from build123d import *

# Parameters (mm, degrees)
F0_W     = 101.6
F0_H     = 152.4
F0_H_2   = 101.6
F1_DEPTH = 152.4
F2_W     = 101.6
F2_H     = 101.6
F3_DEPTH = 228.601
F4_R     = 25.4
F5_DEPTH = 152.401


with BuildPart() as f1:
    # F0 (on Top) → F1 (new body)
    with BuildSketch(Plane.XY):
        with Locations((50.8, 76.2)):
            Rectangle(F0_W, F0_H)
        with Locations((50.8, -50.8)):
            Rectangle(F0_W, F0_H_2)
        Polygon((-76.2, 254), (0, 152.4), (101.6, 152.4), (25.4, 254), align=None)
        Polygon((-127, 304.8), (-76.2, 254), (25.4, 254), align=None)
    extrude(amount=F1_DEPTH)

    # F2 (on face) → F3 (cut, through all)
    with BuildSketch(Plane.YZ.offset(101.6)):
        with Locations((-50.8, 76.2)):
            Rectangle(F2_W, F2_H)
    extrude(amount=-F3_DEPTH, mode=Mode.SUBTRACT)

    # F4 (on face) → F5 (cut, through all)
    with BuildSketch(Plane.XY.offset(152.4)):
        with Locations((50.8, -50.8)):
            Circle(F4_R)
        with BuildLine():
            ThreePointArc((101.6, -50.8), (86.721024, -86.721024), (50.8, -101.6))
            Line((50.8, -101.6), (101.6, -101.6))
            Line((101.6, -101.6), (101.6, -50.8))
        make_face()
        with BuildLine():
            ThreePointArc((50.8, -101.6), (14.878976, -86.721024), (0, -50.8))
            Line((0, -50.8), (0, -101.6))
            Line((0, -101.6), (50.8, -101.6))
        make_face()
    extrude(amount=-F5_DEPTH, mode=Mode.SUBTRACT)


solid = f1.part
Source: CAD feature listing. Evaluate the final solid. Frame: model axes, mm. A direction names the side the tool comes from. Give positions to 0.01 mm unless a question says otherwise; leave off trailing zeros. Write each loop counter-clockwise with the first axis right and the second up, starting at its lowest first coordinate (ties: lowest second). Pieces come first, ordered by that corner, then holes. Notation, with made-up numbers: M -24,88 L -2,88 A12 cw -2,97 Z; hole C 3,-1 d4. An arc over 180 degrees is marked long. Return JSON: item names as keys, results as strings. Group by question number.
1) Cut plane A-A, the plane z = 131. Output: boundary loops of the cut face in (x, y).
2) First-contact query: pin 1 Ø8 at (x, z) = (19, 86.5) entering from -Y; pin 2 Ø12 at (x, z) = (-69, 92) entering from +Y; pin 3 Ø1.5 at (y, z) = (88, 19) entering from -X. Flat tips, straight axial feed; report the tip coordinate or a pass-through.
3) Ray query, L1, parallel to X at y = -50, z = 5; L2, parallel to X at y = 118.5, z = 83.5; L3, parallel to Y at x = 50.8, z = 140. Return the intervals inside material, ascending.
4) Set-up query: faces 1 (the face through (0, 75, 75)), 2 (the face through (101.6, 72, 75)), 3 (the face through (52, 0, 75)). Return all of +Z, -Z, +X, -X, +Y, -Y with unobstructed straight access to the full face (end or side cutting, diameter ignored); none if empty.
5) Draft query along Z for faces 4 (the face through (74, -40, 25.4)), 5 (the face through (36, 104, 0)), 6 (the face through (74, -40, 127)), 7 (the face through (30.643, -66.256, 139.878)). Return one class per face: released by +Z, released by -Z, zero draft, split by the parting line, or undercut.
6) Cut plane C-C, the plane x = -97. Output: boundary loops of the cut face in (y, z), then the cut area to 3 significant figures.
7) Cut plane B-B, the plane z = 44. Output: boundary loops of the cut face in (x, y), then the cut area to 3 significant figures.
8) Cut plane D-D, the plane y = 115. Output: boundary loops of the cut face in (x, z).
Data:
{
 "1": {"outline": "M -127,304.8 L -76.2,254 L 0,152.4 L 0,-50.8 A50.8 ccw 50.8,-101.6 A50.8 ccw 101.6,-50.8 L 101.6,152.4 L 25.4,254 Z; hole C 50.8,-50.8 d50.8"},
 "2": {"pin 1": "stops at y = 0", "pin 2": "stops at y = 287.47", "pin 3": "stops at x = 0"},
 "3": {"L1": "x = 0 to 25.41, 76.19 to 101.6", "L2": "x = 0 to 101.6", "L3": "y = -101.6 to -76.2, -25.4 to 220.13"},
 "4": {"face 1": "+Z, -Z, -X, -Y", "face 2": "+Z, -Z, +X, +Y, -Y", "face 3": "+X, -X, -Y"},
 "5": {"face 4": "undercut", "face 5": "released by -Z", "face 6": "undercut", "face 7": "zero draft"},
 "6": {"outline": "M 274.8,0 L 294.8,0 L 294.8,152.4 L 274.8,152.4 Z", "area": "3,050 mm²"},
 "7": {"outline": "M -127,304.8 L -76.2,254 L 0,152.4 L 0,0 L 101.6,0 L 101.6,152.4 L 25.4,254 Z", "area": "28,400 mm²"},
 "8": {"outline": "M 0,0 L 101.6,0 L 101.6,152.4 L 0,152.4 Z"}
}
